```python
from build123d import *

# Parameters (mm, degrees)
SKETCH1_W           = 12.7
SKETCH1_H           = 50.8
BOSS_EXTRUDE1_DEPTH = 50.8
SKETCH2_R           = 3.2639
CUT_EXTRUDE1_DEPTH  = 19.05
SKETCH3_W           = 33.02
SKETCH3_H           = 29.21
CUT_EXTRUDE2_DEPTH  = 13.7
FILLET1_R           = 10.16


with BuildPart() as part:
    # Sketch1 → Boss-Extrude1 (new body)
    with BuildSketch(Plane.XY):
        with Locations((6.35, 25.4)):
            Rectangle(SKETCH1_W, SKETCH1_H)
    extrude(amount=BOSS_EXTRUDE1_DEPTH)

    # Sketch2 → Cut-Extrude1 (cut)
    with BuildSketch(Plane.XY.offset(50.8)):
        with Locations((6.35, 44.45)):
            Circle(SKETCH2_R)
        with Locations((6.35, 6.35)):
            Circle(SKETCH2_R)
    cut_extrude1 = extrude(amount=-CUT_EXTRUDE1_DEPTH, mode=Mode.SUBTRACT)

    # Mirror1: Cut-Extrude1 across plane
    add(cut_extrude1.mirror(Plane.XY.offset(25.4)), mode=Mode.SUBTRACT)

    # Sketch3 → Cut-Extrude2 (cut, through all)
    with BuildSketch(Plane.ZY):
        with Locations((25.4, 25.4)):
            Rectangle(SKETCH3_W, SKETCH3_H)
    extrude(amount=-CUT_EXTRUDE2_DEPTH, mode=Mode.SUBTRACT)

    # Fillet1
    fillet1_edges = [part.edges().sort_by_distance(p)[0] for p in [
        (6.35, 10.795, 8.89),
        (6.35, 40.005, 8.89),
        (6.35, 40.005, 41.91),
        (6.35, 10.795, 41.91),
    ]]
    fillet(fillet1_edges, radius=FILLET1_R)


solid = part.part
```
The listing builds one solid part. Answer for the finished solid, in the listing's coordinates (mm). A direction names the side the tool comes from. Round coordinates to 2 decimals unless told otherwise and drop trailing zeros. Loops run counter-clockwise (first coordinate to the right, second up) from the corner with the lowest first, then second, coordinate; pieces in that order, holes last. Notation, with made-up numbers: (58, 26) - (80, 26) arc R5 ccw to (80, 34) - close; hole circle Ø9 at (58, 9). An arc over 180 degrees is marked (long way). Return JSON: item names as keys, results as strings. Group by question number.
1. The part is cut by section A-A on y = 26. Determine the outline of the cut face in (x, z), then the cut area to 3 significant figures.
2. The part is cut by section B-B on z = 30. Determine the outline of the cut face in (x, y) (3 decimals), then the cut area to 3 significant figures.
3. The mould has two halves that part along X. Classify faces 4 (the flat face through (6, 26, 50.8)), 5 (the flat face through (12.7, 25, 8)), 6 (the flat face through (6, 44, 31.75)): pulls with the +X half, pulls with the -X half, needs draft (parallel to the pull), parting line crosses it, or undercut.
4. The part is cut by section C-C on x = 1. Determine the outline of the cut face in (y, z) (3 decimals), then the cut area to 3 significant figures.
5. Each of these flat-tipped pins is pushed along its axis until it touches: P1, Ø6, axis at x = 6.35, y = 44.45, coming from the +Z side; P2, Ø3.5, axis at x = 7, y = 7, coming from the -Z side. Where does it stop, or does it pass through?
6. The part is cut by section D-D on z = 47. Determine the outline of the cut face in (x, y).
7. Consider probe 1 along Y at (x, z) = (6.35, 4.5); probe 2 along Z at (x, y) = (8, 26); probe 3 along Y at (x, z) = (5.75, 41). Determine where each line is inside the solid, lowest interval first.
8. Which of the six approach directions +Z, -Z, +X, -X, +Y, -Y give full straight-line access (tool end or side, diameter ignored) to faces 1 (the cylindrical face through (5.925, 47.686, 9.392)), 2 (the cylindrical face through (5.925, 47.686, 41.408)), 3 (the cylindrical face through (6.44, 36.95, 39.01))?
Resolved:
{
 "1": {"outline": "(0, 0) - (12.7, 0) - (12.7, 8.89) - (0, 8.89) - close; (0, 41.91) - (12.7, 41.91) - (12.7, 50.8) - (0, 50.8) - close", "area": "226 mm²"},
 "2": {"outline": "(0, 0) - (12.7, 0) - (12.7, 10.795) - (0, 10.795) - close; (0, 40.005) - (12.7, 40.005) - (12.7, 50.8) - (0, 50.8) - close", "area": "274 mm²"},
 "3": {"face 4": "needs draft", "face 5": "pulls with the +X half", "face 6": "undercut"},
 "4": {"outline": "(0, 0) - (50.8, 0) - (50.8, 50.8) - (0, 50.8) - close; hole (10.795, 19.05) arc R10.16 ccw to (20.955, 8.89) - (29.845, 8.89) arc R10.16 ccw to (40.005, 19.05) - (40.005, 31.75) arc R10.16 ccw to (29.845, 41.91) - (20.955, 41.91) arc R10.16 ccw to (10.795, 31.75) - close", "area": "1,700 mm²"},
 "5": {"P1": "stops at z = 31.75", "P2": "stops at z = 19.05"},
 "6": {"outline": "(0, 0) - (12.7, 0) - (12.7, 50.8) - (0, 50.8) - close; hole circle Ø6.53 at (6.35, 6.35); hole circle Ø6.53 at (6.35, 44.45)"},
 "7": {"probe 1": "y = 0 to 3.09, 9.61 to 41.19, 47.71 to 50.8", "probe 2": "z = 0 to 8.89, 41.91 to 50.8", "probe 3": "y = 0 to 3.14, 9.56 to 16.75, 34.05 to 41.24, 47.66 to 50.8"},
 "8": {"face 1": "-Z", "face 2": "+Z", "face 3": "+X, -X"}
}
